Here's how the part is built. I have some questions about the finished solid (model axes, mm). Face numbers are marked on the shaded views. A direction names the side the tool comes from. Coordinates: 2 decimals unless noted, no trailing zeros. Write each loop counter-clockwise with the first axis right and the second up, starting at its lowest first coordinate (ties: lowest second). Pieces come first, ordered by that corner, then holes.
(1) Please list where these lines run through material, in increasing order: probe 1 along Y at (x, z) = (10.95, 0.65); probe 2 along Y at (x, z) = (2.5, 3.5); probe 3 along Z at (x, y) = (0.5, 9.5).
(2) Which directions (+Z, -Z, +X, -X, +Y, -Y) give clear straight access to the entire face, cutting with the end or side of a thin tool? Please do the marked faces 1 and 2.
(3) For pin 1 Ø5 at (y, z) = (3.5, 4.5) entering from -X; pin 2 Ø1 at (x, y) = (8.5, 2.5) entering from -Z; pin 3 Ø1.2 at (y, z) = (-10.5, 3) entering from +X; pin 4 Ø3 at (y, z) = (-8, 1.5) entering from -X, each with a flat end and sliding along its axis, tell me the tip position at first contact or that it passes through.
(4) Imagine slicing it at A-A, the plane x = 0. List the corners of the cut face in (y, z) for me.
(5) Imagine slicing it at D-D, the plane y = -11. List the corners of the cut face in (x, z) for me.
(6) Imagine slicing it at C-C, the plane x = -3.75. List the corners of the cut face in (y, z) for me.
(7) Thinking about a two-plate mould opening in Y: for the marked faces 3, 4, 5 and 6, which applies, released by +Y, released by -Y, zero draft, split by the parting line, or undercut?
(8) Imagine slicing it at B-B, the plane y = 11.3. List the corners of the cut face in (x, z) for me, plus the area to 3 significant figures.
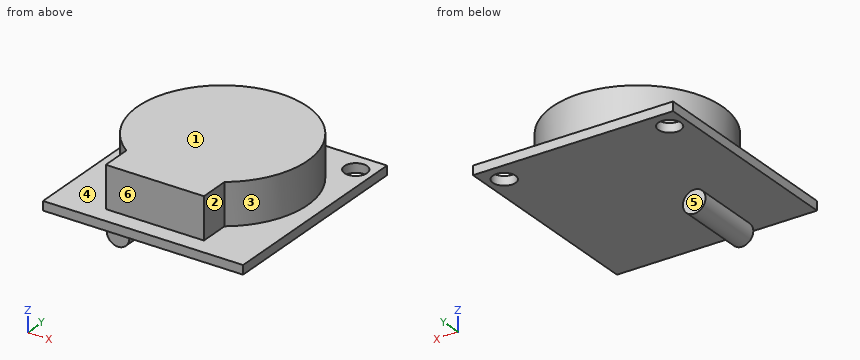
```python
from build123d import *

# Parameters (mm, degrees)
F0_W     = 26.5
F0_H     = 28
F0_R     = 1.5
F1_DEPTH = 1.2
F3_DEPTH = 5.5
F4_R     = 1.5
F5_DEPTH = 9.3


with BuildPart() as f1:
    # F0 (on Top) → F1 (new body)
    with BuildSketch(Plane.XY):
        Rectangle(F0_W, F0_H)
        with Locations((-10.95, 11.3)):
            Circle(F0_R, mode=Mode.SUBTRACT)
        with Locations((10.95, 11.3)):
            Circle(F0_R, mode=Mode.SUBTRACT)
    extrude(amount=F1_DEPTH)

    # F2 (on face) → F3 (join)
    with BuildSketch(Plane.XY.offset(1.2)):
        with BuildLine():
            Line((6.5, -11.7), (6.5, -7.7))
            ThreePointArc((6.5, -7.7), (0, 12.7321838361), (-6.5, -7.7))
            Line((-6.5, -7.7), (-6.5, -11.7))
            Line((-6.5, -11.7), (6.5, -11.7))
        make_face()
    extrude(amount=F3_DEPTH)

    # F4 (on face) → F5 (join)
    with BuildSketch(Plane.XZ.offset(11.7)):
        with Locations((-4.8800413497, -1.49)):
            Circle(F4_R)
    extrude(amount=-F5_DEPTH)


solid = f1.part
```
Recorded:
1. probe 1: y = -14 to 9.8, 12.8 to 14
1. probe 2: y = -11.7 to 12.45
1. probe 3: z = 0 to 6.7
2. face 1: +Z, +X, -X, +Y, -Y
2. face 2: +Z, +X, -Y
3. pin 1: stops at x = -11.25
3. pin 2: stops at z = 0
3. pin 3: stops at x = 6.5
3. pin 4: stops at x = -13.25
4. outline: (-14, 0) - (14, 0) - (14, 1.2) - (12.73, 1.2) - (12.73, 6.7) - (-11.7, 6.7) - (-11.7, 1.2) - (-14, 1.2) - close
5. outline: (-13.25, 0) - (-5.05, 0) arc R1.5 ccw (long way) to (-4.71, 0) - (13.25, 0) - (13.25, 1.2) - (6.5, 1.2) - (6.5, 6.7) - (-6.5, 6.7) - (-6.5, 1.2) - (-13.25, 1.2) - close
6. outline: (-14, 0) - (14, 0) - (14, 1.2) - (12.09, 1.2) - (12.09, 6.7) - (-11.7, 6.7) - (-11.7, 1.2) - (-14, 1.2) - close; (-11.7, -2.48) - (-2.4, -2.48) - (-2.4, -0.5) - (-11.7, -0.5) - close
7. face 3: split by the parting line
7. face 4: zero draft
7. face 5: released by +Y
7. face 6: released by -Y
8. outline: (-13.25, 0) - (-12.45, 0) - (-12.45, 1.2) - (-13.25, 1.2) - close; (-9.45, 0) - (9.45, 0) - (9.45, 1.2) - (5.49, 1.2) - (5.49, 6.7) - (-5.49, 6.7) - (-5.49, 1.2) - (-9.45, 1.2) - close; (12.45, 0) - (13.25, 0) - (13.25, 1.2) - (12.45, 1.2) - close
8. area: 85.0 mm2
